The model under review builds one solid part; all positions refer to its coordinate system, in mm. Give positions to 0.01 mm unless a question says otherwise; leave off trailing zeros. Loops run counter-clockwise (first coordinate to the right, second up) from the corner with the lowest first, then second, coordinate; pieces in that order, holes last. Notation, with made-up numbers: M -27.75,46.5 L 6.25,46.5 A23 ccw 6.25,64.5 Z; hole C -9.5,70 d3. An arc over 180 degrees is marked long. Write item = value, one per line. Start each with the question number.
1. We need section B-B on y = 0.8. Count the separate pieces of the cut face and the enclosed holes in it, then the cut area to 3 significant figures.
2. Wall thickness on line 1 along Z through (x, y) = (6.5, 0.9); line 2 along X through (y, z) = (0.5, 40); line 3 along Z through (x, y) = (2, 1.1): over which ranges is each line inside the solid? List them lowest first. Write a range as from..to.
3. We need section A-A on z = 36.5. Give the boundary of the cut face in (x, y).
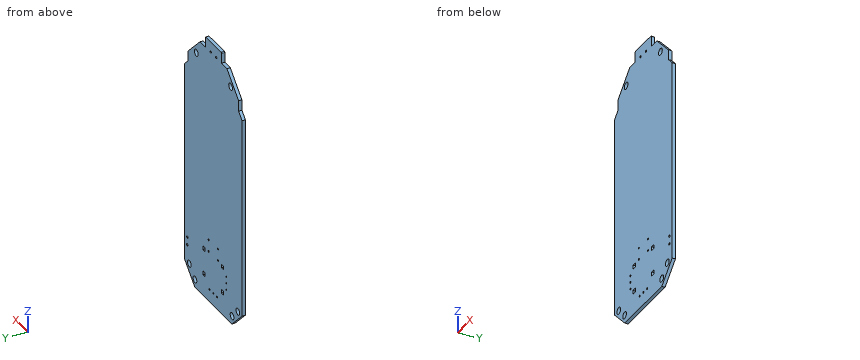
Autodesk Inventor part; units mm, degrees
ref_plane "Work Plane1" through (0, 0.615, 0) normal (0, 1, 0) x (1, 0, 0)
ref_plane "Work Plane3" through (0.0314, 0, 32.2255) normal (1, 0, 0) x (0, 0, -1)
ref_plane "Work Plane5" through (12.6739, 1.23, -50.7145) normal (0, 0.766, -0.6428) x (-1, 0, 0)
sketch "Sketch1" plane through (0, 0, 0) normal (0, 1, 0) x (-1, 0, 0)
  line L0 (5.5496, 46.5995) -> (5.5496, 50.3655)
  arc A0 (5.5496, 50.3655) -> (5.2006, 50.7145) centre (5.2006, 50.3655) ccw
  line L1 (5.2006, 50.7145) -> (-5.2234, 50.7145)
  arc A1 (-5.2234, 50.7145) -> (-5.4614, 50.4765) centre (-5.2234, 50.4765) ccw
  line L2 (-5.4614, 50.4765) -> (-5.4614, 46.5995)
  line L3 (-5.4614, 46.5995) -> (-9.2444, 46.5995)
  line L4 (-9.2444, 46.5995) -> (-17.2394, 38.6045)
  line L5 (-17.2394, 38.6045) -> (-17.2394, 34.8415)
  line L6 (-17.2394, 34.8415) -> (-19.7395, 32.2255)
  line L7 (-19.7395, 32.2255) -> (-19.7395, -43.6601)
  line L8 (-19.7395, -43.6601) -> (-12.6739, -50.7145)
  line L9 (-12.6739, -50.7145) -> (12.6966, -50.7145)
  line L10 (12.6966, -50.7145) -> (19.6766, -43.7345)
  line L11 (19.6766, -43.7345) -> (19.6766, 32.1505)
  line L12 (19.6766, 32.1505) -> (17.2796, 34.5475)
  line L13 (17.2796, 34.5475) -> (17.2796, 38.6115)
  line L14 (17.2796, 38.6115) -> (9.2916, 46.5995)
  line L15 (9.2916, 46.5995) -> (5.5496, 46.5995)
  circle A2 centre (12.7766, -47.6345) radius 1.27
  circle A3 centre (-12.6044, -47.6345) radius 1.27
  circle A4 centre (16.7766, -43.6345) radius 1.27
  circle A5 centre (-16.4774, -43.6345) radius 1.27
  circle A6 centre (11.7766, 40.9591) radius 1.27
  circle A7 centre (-11.7154, 40.9591) radius 1.27
  circle A8 centre (-1.8694, 46.7845) radius 0.425
  circle A9 centre (1.9306, 46.7845) radius 0.425
  circle A10 centre (-17.8584, -37.1345) radius 0.45
  circle A11 centre (-17.8584, -34.1345) radius 0.45
  arc A12 (3.4251, -26.9975) -> (2.7461, -26.9975) centre (3.0856, -26.9975) ccw
  arc A13 (2.7461, -26.9975) -> (3.4251, -26.9975) centre (3.0856, -26.9975) ccw
  arc A14 (3.4251, -26.9975) -> (2.7461, -26.9975) centre (3.0856, -26.9975) ccw
  arc A15 (2.7461, -26.9975) -> (3.4251, -26.9975) centre (3.0856, -26.9975) ccw
  arc A16 (3.4251, -31.4425) -> (2.7461, -31.4425) centre (3.0856, -31.4425) ccw
  arc A17 (2.7461, -31.4425) -> (3.4251, -31.4425) centre (3.0856, -31.4425) ccw
  arc A18 (3.4251, -31.4425) -> (2.7461, -31.4425) centre (3.0856, -31.4425) ccw
  arc A19 (2.7461, -31.4425) -> (3.4251, -31.4425) centre (3.0856, -31.4425) ccw
  arc A20 (-2.9249, -31.4425) -> (-3.6039, -31.4425) centre (-3.2644, -31.4425) ccw
  arc A21 (-3.6039, -31.4425) -> (-2.9249, -31.4425) centre (-3.2644, -31.4425) ccw
  arc A22 (-2.9249, -31.4425) -> (-3.6039, -31.4425) centre (-3.2644, -31.4425) ccw
  arc A23 (-3.6039, -31.4425) -> (-2.9249, -31.4425) centre (-3.2644, -31.4425) ccw
  arc A24 (-2.9249, -26.9975) -> (-3.6039, -26.9975) centre (-3.2644, -26.9975) ccw
  arc A25 (-3.6039, -26.9975) -> (-2.9249, -26.9975) centre (-3.2644, -26.9975) ccw
  arc A26 (-2.9249, -26.9975) -> (-3.6039, -26.9975) centre (-3.2644, -26.9975) ccw
  arc A27 (-3.6039, -26.9975) -> (-2.9249, -26.9975) centre (-3.2644, -26.9975) ccw
  line L16 (7.0146, -32.9585) -> (7.0146, -31.4505)
  line L17 (7.0146, -31.4505) -> (5.5066, -31.4505)
  line L18 (5.5066, -31.4505) -> (5.5066, -32.9585)
  line L19 (5.5066, -32.9585) -> (7.0146, -32.9585)
  line L20 (7.0146, -32.9585) -> (7.0146, -31.4505)
  line L21 (7.0146, -31.4505) -> (5.5066, -31.4505)
  line L22 (5.5066, -31.4505) -> (5.5066, -32.9585)
  line L23 (5.5066, -32.9585) -> (7.0146, -32.9585)
  line L24 (7.0146, -42.7375) -> (7.0146, -41.2295)
  line L25 (7.0146, -41.2295) -> (5.5066, -41.2295)
  line L26 (5.5066, -41.2295) -> (5.5066, -42.7375)
  line L27 (5.5066, -42.7375) -> (7.0146, -42.7375)
  line L28 (7.0146, -42.7375) -> (7.0146, -41.2295)
  line L29 (7.0146, -41.2295) -> (5.5066, -41.2295)
  line L30 (5.5066, -41.2295) -> (5.5066, -42.7375)
  line L31 (5.5066, -42.7375) -> (7.0146, -42.7375)
  line L32 (-5.6854, -42.7375) -> (-5.6854, -41.2295)
  line L33 (-5.6854, -41.2295) -> (-7.1934, -41.2295)
  line L34 (-7.1934, -41.2295) -> (-7.1934, -42.7375)
  line L35 (-7.1934, -42.7375) -> (-5.6854, -42.7375)
  line L36 (-5.6854, -42.7375) -> (-5.6854, -41.2295)
  line L37 (-5.6854, -41.2295) -> (-7.1934, -41.2295)
  line L38 (-7.1934, -41.2295) -> (-7.1934, -42.7375)
  line L39 (-7.1934, -42.7375) -> (-5.6854, -42.7375)
  line L40 (-5.6854, -32.9585) -> (-5.6854, -31.4505)
  line L41 (-5.6854, -31.4505) -> (-7.1934, -31.4505)
  line L42 (-7.1934, -31.4505) -> (-7.1934, -32.9585)
  line L43 (-7.1934, -32.9585) -> (-5.6854, -32.9585)
  line L44 (-5.6854, -32.9585) -> (-5.6854, -31.4505)
  line L45 (-5.6854, -31.4505) -> (-7.1934, -31.4505)
  line L46 (-7.1934, -31.4505) -> (-7.1934, -32.9585)
  line L47 (-7.1934, -32.9585) -> (-5.6854, -32.9585)
  arc A28 (9.1401, -34.554) -> (8.4611, -34.554) centre (8.8006, -34.554) ccw
  arc A29 (8.4611, -34.554) -> (9.1401, -34.554) centre (8.8006, -34.554) ccw
  arc A30 (9.1401, -34.554) -> (8.4611, -34.554) centre (8.8006, -34.554) ccw
  arc A31 (8.4611, -34.554) -> (9.1401, -34.554) centre (8.8006, -34.554) ccw
  arc A32 (9.1401, -39.634) -> (8.4611, -39.634) centre (8.8006, -39.634) ccw
  arc A33 (8.4611, -39.634) -> (9.1401, -39.634) centre (8.8006, -39.634) ccw
  arc A34 (9.1401, -39.634) -> (8.4611, -39.634) centre (8.8006, -39.634) ccw
  arc A35 (8.4611, -39.634) -> (9.1401, -39.634) centre (8.8006, -39.634) ccw
  arc A36 (9.1401, -37.094) -> (8.4611, -37.094) centre (8.8006, -37.094) ccw
  arc A37 (8.4611, -37.094) -> (9.1401, -37.094) centre (8.8006, -37.094) ccw
  arc A38 (9.1401, -37.094) -> (8.4611, -37.094) centre (8.8006, -37.094) ccw
  arc A39 (8.4611, -37.094) -> (9.1401, -37.094) centre (8.8006, -37.094) ccw
  arc A40 (2.7901, -45.984) -> (2.1111, -45.984) centre (2.4506, -45.984) ccw
  arc A41 (2.1111, -45.984) -> (2.7901, -45.984) centre (2.4506, -45.984) ccw
  arc A42 (2.7901, -45.984) -> (2.1111, -45.984) centre (2.4506, -45.984) ccw
  arc A43 (2.1111, -45.984) -> (2.7901, -45.984) centre (2.4506, -45.984) ccw
  arc A44 (-2.2899, -45.984) -> (-2.9689, -45.984) centre (-2.6294, -45.984) ccw
  arc A45 (-2.9689, -45.984) -> (-2.2899, -45.984) centre (-2.6294, -45.984) ccw
  arc A46 (-2.2899, -45.984) -> (-2.9689, -45.984) centre (-2.6294, -45.984) ccw
  arc A47 (-2.9689, -45.984) -> (-2.2899, -45.984) centre (-2.6294, -45.984) ccw
  arc A48 (0.2501, -45.984) -> (-0.4289, -45.984) centre (-0.0894, -45.984) ccw
  arc A49 (-0.4289, -45.984) -> (0.2501, -45.984) centre (-0.0894, -45.984) ccw
  arc A50 (0.2501, -45.984) -> (-0.4289, -45.984) centre (-0.0894, -45.984) ccw
  arc A51 (-0.4289, -45.984) -> (0.2501, -45.984) centre (-0.0894, -45.984) ccw
  point P0 (5.5496, 50.3655)
  point P1 (-0.4289, -45.984)
  point P2 (0.2501, -45.984)
  point P3 (2.1111, -45.984)
  point P4 (2.7901, -45.984)
  point P5 (8.4611, -39.634)
  point P6 (9.1401, -39.634)
  point P7 (-3.6039, -26.9975)
  point P8 (-2.9249, -26.9975)
  point P9 (2.7461, -31.4425)
  point P10 (3.4251, -31.4425)
  point P11 (2.7461, -26.9975)
  point P12 (3.4251, -26.9975)
  point P13 (-3.6039, -31.4425)
  point P14 (-2.9249, -31.4425)
  point P15 (8.4611, -34.554)
  point P16 (9.1401, -34.554)
  point P17 (8.4611, -37.094)
  point P18 (9.1401, -37.094)
  point P19 (-2.9689, -45.984)
  point P20 (-2.2899, -45.984)
extrude "Extrusion1" add sketch "Sketch1" along normal blind 1.23
ref_plane "Work Plane1" through (0, 0.615, 0) normal (0, 1, 0) x (1, 0, 0)
ref_plane "Work Plane3" through (0.0314, 0, 32.2255) normal (1, 0, 0) x (0, 0, -1)
ref_plane "Work Plane5" through (12.6739, 1.23, -50.7145) normal (0, 0.766, -0.6428) x (-1, 0, 0)
ref_plane "Work Plane6" through (-5.2006, 0, 0) normal (0, 0, 1) x (1, 0, 0)
sketch "Sketch3" plane through (0, 1.23, 0) normal (0, 1, 0) x (1, 0, 0)
  circle A0 centre (17.8584, 37.1345) radius 0.45
  circle A1 centre (17.8584, 34.1345) radius 0.45
  line L0 (17.8584, 37.1345) -> (17.8584, 34.1345)
  line L1 (17.8584, 35.6345) -> (19.3564, 35.6345)
  line L2 (19.7395, -32.2255) -> (19.7395, 43.6601)
ref_plane "Work Plane7" through (17.8584, 1.23, -35.6345) normal (0, 0, 1) x (1, 0, 0)
properties part number "PCB"
Final values:
q1.separate_pieces = 1
q1.enclosed_holes = 24
q1.area = 3,660 mm²
q2.line_1 = -50.71..-42.74, -41.23..-32.96, -31.45..46.6
q2.line_2 = -15.89..-12.61, -10.94..10.88, 12.55..15.84
q2.line_3 = -50.71..46.38, 47.19..50.71
q3.outline = M -17.28,0 L 17.24,0 L 17.24,1.23 L -17.28,1.23 Z
